Verification items for the finished model (mm, model axes). Face numbers are marked on the shaded views. A direction names the side the tool comes from. Round coordinates to 2 decimals unless told otherwise and drop trailing zeros. Loops run counter-clockwise (first coordinate to the right, second up) from the corner with the lowest first, then second, coordinate; pieces in that order, holes last. Notation, with made-up numbers: (7, 24.5) -> (27, 24.5) arc R8 cw to (27, 31.5) -> close; hole circle Ø7 at (-7, 70.5). An arc over 180 degrees is marked (long way). Use CSV: the item, a comma, the result in double quotes. Start each with the question number.
```python
from build123d import *

# Parameters (mm, degrees)
SKETCH1_R           = 152.4
BOSS_EXTRUDE1_DEPTH = 10
SKETCH2_W           = 25.4
SKETCH2_H           = 25.4
SKETCH2_W_2         = 22.225
SKETCH2_H_2         = 22.225
BOSS_EXTRUDE2_DEPTH = 30


with BuildPart() as part:
    # Sketch1 → Boss-Extrude1 (new body)
    with BuildSketch(Plane.XY):
        Circle(SKETCH1_R)
    extrude(amount=BOSS_EXTRUDE1_DEPTH)

    # Sketch2 → Boss-Extrude2 (add)
    # profile 1 of 2: a face of its own
    with BuildSketch(Plane.XY.offset(10)):
        Rectangle(SKETCH2_W, SKETCH2_H)
        Rectangle(SKETCH2_W_2, SKETCH2_H_2, mode=Mode.SUBTRACT)
    # profile 2 of 2: a face of its own
    with BuildSketch(Plane.XY.offset(10)):
        with Locations((0, 120)):
            Rectangle(SKETCH2_W, SKETCH2_H)
        with Locations((0, 120)):
            Rectangle(SKETCH2_W_2, SKETCH2_H_2, mode=Mode.SUBTRACT)
    extrude(amount=BOSS_EXTRUDE2_DEPTH)


solid = part.part
```
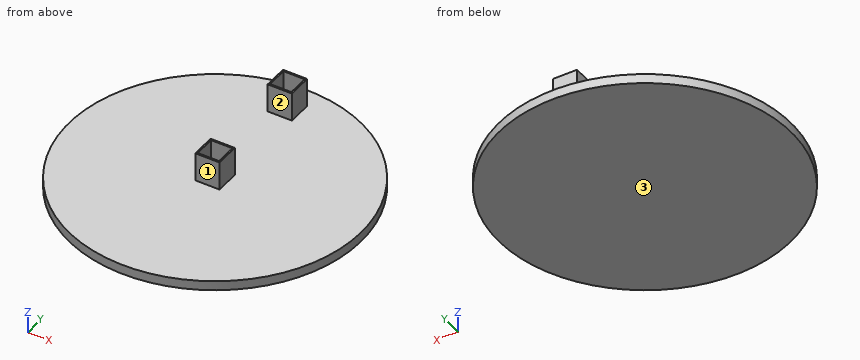
Q1. Thickness scan on L1, parallel to Y at x = 3.5, z = 34.5; L2, parallel to X at y = 111.5, z = 31; L3, parallel to Z at x = 56.5, y = 41.5. Record the ranges inside material, lowest first. Write a range as from..to.
Q2. Cross-section at C-C (y = 0). Record the boundary of the cut face in (x, z), and give its area (3 significant figures).
Q3. Cross-section at A-A (z = 32.5). Record the boundary of the cut face in (x, y).
Q4. Tool access check on the marked faces 1, 2 and 3. Record the directions out of +Z, -Z, +X, -X, +Y, -Y that give a thin tool (end or side, any length) a straight path to the whole face; none if there is none.
Q5. Depth check by flat-ended pin: pin 1 Ø1.5 at (x, y) = (34, 32.5) entering from +Z; pin 2 Ø12.5 at (y, z) = (-1.5, 30) entering from -X; pin 3 Ø1.5 at (x, y) = (26.5, -107.5) entering from -Z; pin 4 Ø12 at (y, z) = (109, 29) entering from +X. Enter the tip coordinate at first touch or a pass-through.
Q6. Cross-section at B-B (x = 0). Record the boundary of the cut face in (y, z).
Q7. Cross-section at D-D (y = 112.5). Record the boundary of the cut face in (x, z), and give its area (3 significant figures).
Answer list:
1,L1,"y = -12.7..-11.11, 11.11..12.7, 107.3..108.89, 131.11..132.7"
1,L2,"x = -12.7..-11.11, 11.11..12.7"
1,L3,"z = 0..10"
2,outline,"(-152.4, 0) -> (152.4, 0) -> (152.4, 10) -> (12.7, 10) -> (12.7, 40) -> (11.11, 40) -> (11.11, 10) -> (-11.11, 10) -> (-11.11, 40) -> (-12.7, 40) -> (-12.7, 10) -> (-152.4, 10) -> close"
2,area,"3,140 mm2"
3,outline,"(-12.7, -12.7) -> (12.7, -12.7) -> (12.7, 12.7) -> (-12.7, 12.7) -> close; (-12.7, 107.3) -> (12.7, 107.3) -> (12.7, 132.7) -> (-12.7, 132.7) -> close; hole (-11.11, -11.11) -> (11.11, -11.11) -> (11.11, 11.11) -> (-11.11, 11.11) -> close; hole (-11.11, 108.89) -> (11.11, 108.89) -> (11.11, 131.11) -> (-11.11, 131.11) -> close"
4,face 1,"+Z, +X, -X, -Y"
4,face 2,"+Z, +X, -X"
4,face 3,"-Z, +X, -X, +Y, -Y"
5,pin 1,"stops at z = 10"
5,pin 2,"stops at x = -12.7"
5,pin 3,"stops at z = 0"
5,pin 4,"stops at x = 12.7"
6,outline,"(-152.4, 0) -> (152.4, 0) -> (152.4, 10) -> (132.7, 10) -> (132.7, 40) -> (131.11, 40) -> (131.11, 10) -> (108.89, 10) -> (108.89, 40) -> (107.3, 40) -> (107.3, 10) -> (12.7, 10) -> (12.7, 40) -> (11.11, 40) -> (11.11, 10) -> (-11.11, 10) -> (-11.11, 40) -> (-12.7, 40) -> (-12.7, 10) -> (-152.4, 10) -> close"
7,outline,"(-102.81, 0) -> (102.81, 0) -> (102.81, 10) -> (12.7, 10) -> (12.7, 40) -> (11.11, 40) -> (11.11, 10) -> (-11.11, 10) -> (-11.11, 40) -> (-12.7, 40) -> (-12.7, 10) -> (-102.81, 10) -> close"
7,area,"2,150 mm2"
